Here's how the part is built. I have some questions about the finished solid (model axes, mm). Face numbers are marked on the shaded views. Round coordinates to 2 decimals unless told otherwise and drop trailing zeros. Write each loop counter-clockwise with the first axis right and the second up, starting at its lowest first coordinate (ties: lowest second). Pieces come first, ordered by that corner, then holes. Notation, with made-up numbers: (19, 51.25) -> (49, 51.25) arc R22 ccw to (49, 67.25) -> close; hole circle Ø8 at (69, -26). An arc over 180 degrees is marked (long way). Answer as CSV lines item,"result".
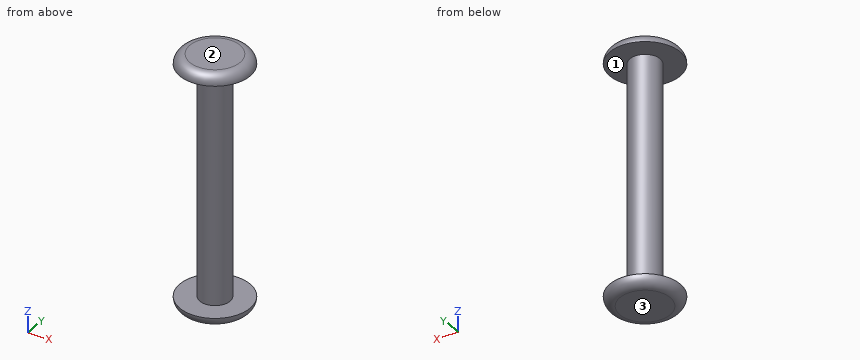
```python
from build123d import *

# Parameters (mm, degrees)
SKETCH1_R           = 3.75
BOSS_EXTRUDE1_DEPTH = 28.75
BOSS_EXTRUDE2_START = 2.5
SKETCH2_R           = 8.75
SKETCH2_R_2         = 3.75
BOSS_EXTRUDE2_DEPTH = 2.5
SKETCH3_R           = 8.75
BOSS_EXTRUDE3_DEPTH = 2.5
FILLET1_R           = 2.5


with BuildPart() as part:
    # Sketch1 → Boss-Extrude1 (new, symmetric)
    with BuildSketch(Plane.XY):
        Circle(SKETCH1_R)
    extrude(amount=BOSS_EXTRUDE1_DEPTH, both=True)

    # Sketch2 → Boss-Extrude2 (add)
    # profile 1 of 2: a face of its own
    with BuildSketch(Plane.XY.offset(28.75).offset(BOSS_EXTRUDE2_START)):
        Circle(SKETCH2_R)
        Circle(SKETCH2_R_2, mode=Mode.SUBTRACT)
    # profile 2 of 2: a face of its own
    with BuildSketch(Plane.XY.offset(28.75).offset(BOSS_EXTRUDE2_START)):
        Circle(SKETCH2_R_2)
    extrude(amount=-BOSS_EXTRUDE2_DEPTH)

    # Sketch3 → Boss-Extrude3 (add)
    with BuildSketch(Plane(origin=(0, 0, -28.75), x_dir=(-1, 0, 0), z_dir=(0, 0, -1))):
        with Locations(Location((0, 0, 0), (0, 0, 180))):
            Circle(SKETCH3_R)
    extrude(amount=BOSS_EXTRUDE3_DEPTH)

    # Fillet1
    fillet1_edges = [part.edges().sort_by_distance(p)[0] for p in [
        (-8.75, 0, -31.25),
        (-8.75, 0, 31.25),
    ]]
    fillet(fillet1_edges, radius=FILLET1_R - 0.0001)  # a hair under: the kernel refuses the full size


solid = part.part
```
1. For pin 1 Ø1.5 at (y, z) = (2.5, 12.5) entering from +X; pin 2 Ø1.5 at (x, z) = (-3.5, -12) entering from -Y; pin 3 Ø8 at (x, z) = (-4.5, 12) entering from +Y, each with a flat end and sliding along its axis, tell me the tip position at first contact or that it passes through.
Numbers:
pin 1,"stops at x = 3.32"
pin 2,"stops at y = -2.55"
pin 3,"stops at y = 3.72"
2. If I drill on line 1 (Z direction, x = 4.5, y = 2.5); line 2 (Z direction, x = -3, y = 8); line 3 (X direction, y = 2.25, z = 21.5), over which ranges is the centre line in solid material (lowest first)?
Numbers:
line 1,"z = -31.25 to -28.75, 28.75 to 31.25"
line 2,"z = -29.74 to -28.75, 28.75 to 29.74"
line 3,"x = -3 to 3"
3. If we mould it in two halves opening along Z, with no side actions, what happens to the marked faces 1, 2 and 3? For each: released by +Z, released by -Z, zero draft, split by the parting line, or undercut.
Numbers:
face 1,"undercut"
face 2,"released by +Z"
face 3,"released by -Z"
4. Suppose I cut it at C-C on z = 2. Please give me the cut outline in (x, y), and give its area (3 significant figures).
Numbers:
outline,"circle Ø7.5 at (0, 0)"
area,"44.2 mm^2"
